```python
from build123d import *

# Parameters (mm, degrees)
F0_W     = 9.3324817717
F0_H     = 15.9647651017
F1_DEPTH = 7.62
F2_W     = 2.5024851784
F2_H     = 4.3162275106
F3_DEPTH = 25.4
F4_DEPTH = 25.4
F5_DEPTH = 25.4
F6_W     = 10.77144593
F6_H     = 19.1651917994
F7_DEPTH = 7.62


with BuildPart() as f1:
    # F0 (on Front) → F1 (new body)
    with BuildSketch(Plane.XZ):
        with Locations((-4.6662408859, 29.8102106899)):
            Rectangle(F0_W, F0_H)
    extrude(amount=F1_DEPTH)

    # F2 (on face) → F3 (join)
    with BuildSketch(Plane(origin=(-9.3324817717, 0, 0), x_dir=(0, -1, 0), z_dir=(-1, 0, 0))):
        with Locations((3.4680166282, 23.9859418944)):
            Rectangle(F2_W, F2_H)
    extrude(amount=F3_DEPTH)

    # F4 (add): a face of the model
    f4_faces = [f1.faces().sort_by_distance(p)[0] for p in [
        (-34.7324817717, -3.4680166282, 23.9859418944),
    ]]
    extrude(f4_faces, amount=F4_DEPTH)

    # F5 (add): a face of the model
    f5_faces = [f1.faces().sort_by_distance(p)[0] for p in [
        (-60.1324817717, -3.4680166282, 23.9859418944),
    ]]
    extrude(f5_faces, amount=F5_DEPTH)

    # F6 (on Front) → F7 (join)
    with BuildSketch(Plane.XZ):
        with Locations((-80.5792994797, 30.7407360524)):
            Rectangle(F6_W, F6_H)
    extrude(amount=F7_DEPTH)


solid = f1.part
```
Can you work these out from the model? Positions are in its coordinate system, mm. A direction names the side the tool comes from. Round coordinates to 2 decimals unless told otherwise and drop trailing zeros. Loops run counter-clockwise (first coordinate to the right, second up) from the corner with the lowest first, then second, coordinate; pieces in that order, holes last.
Item 1: Suppose I cut it at D-D, the plane x = -65. Write out the boundary of the cut face in (y, z).
Item 2: Which directions (+Z, -Z, +X, -X, +Y, -Y) give clear straight access to the entire face, cutting with the end or side of a thin tool? Please do faces 1 (the flat face through (-42, -3, 26.144)), 2 (the flat face through (0, -4, 30)), 3 (the flat face through (-42, -4.719, 24)), 4 (the flat face through (-5, -4, 37.793)), 5 (the flat face through (-29, -4, 21.828)).
Item 3: Suppose I cut it at A-A, the plane z = 29.5. Write out the boundary of the cut face in (x, y), then the cut area to 3 significant figures.
Item 4: Suppose I cut it at B-B, the plane y = -1.25. Write out the boundary of the cut face in (x, z), then the cut area to 3 significant figures.
Item 5: Will these pins go through, and if not, where does the flat tip stop? pin 1 Ø4 at (x, y) = (-36, -4) entering from -Z; pin 2 Ø3.5 at (x, z) = (-35, 23.5) entering from -Y; pin 3 Ø2 at (x, y) = (-40.5, -3) entering from +Z.
Item 6: If we mould it in two halves opening along X, with no side actions, what happens to faces 6 (the flat face through (-85.965, -4, 31)), 7 (the flat face through (-81, 0, 31)), 8 (the flat face through (-42, -2.217, 24))? For each: +X half, -X half, draft (parallel to the pull), parting line (faces both ways), or undercut.
Item 7: Please list where these lines run through material, in increasing order: L1, parallel to X at y = -0.75, z = 24.5; L2, parallel to Z at x = -50.5, y = -4; L3, parallel to X at y = -5.25, z = 39.5.
Item 8: Suppose I cut it at C-C, the plane z = 24. Write out the boundary of the cut face in (x, y), then the cut area to 3 significant figures.
Reported:
1. outline: (-4.72, 21.83) - (-2.22, 21.83) - (-2.22, 26.14) - (-4.72, 26.14) - close
2. face 1: +Z, +Y, -Y
2. face 2: +Z, -Z, +X, +Y, -Y
2. face 3: +Z, -Z, -Y
2. face 4: +Z, +X, +Y, -Y
2. face 5: -Z, +X, +Y, -Y
3. outline: (-85.97, -7.62) - (-75.19, -7.62) - (-75.19, 0) - (-85.97, 0) - close; (-9.33, -7.62) - (0, -7.62) - (0, 0) - (-9.33, 0) - close
3. area: 153 mm2
4. outline: (-85.97, 21.16) - (-75.19, 21.16) - (-75.19, 40.32) - (-85.97, 40.32) - close; (-9.33, 21.83) - (0, 21.83) - (0, 37.79) - (-9.33, 37.79) - close
4. area: 355 mm2
5. pin 1: stops at z = 21.83
5. pin 2: stops at y = -4.72
5. pin 3: stops at z = 26.14
6. face 6: -X half
6. face 7: draft
6. face 8: undercut
7. L1: x = -85.97 to -75.19, -9.33 to 0
7. L2: z = 21.83 to 26.14
7. L3: x = -85.97 to -75.19
8. outline: (-85.97, -7.62) - (-75.19, -7.62) - (-75.19, -4.72) - (-9.33, -4.72) - (-9.33, -7.62) - (0, -7.62) - (0, 0) - (-9.33, 0) - (-9.33, -2.22) - (-75.19, -2.22) - (-75.19, 0) - (-85.97, 0) - close
8. area: 318 mm2
